Read the model definition and answer for the solid it produces. Units are mm, in the model's axes. A direction names the side the tool comes from. Coordinates: 2 decimals unless noted, no trailing zeros. Write each loop counter-clockwise with the first axis right and the second up, starting at its lowest first coordinate (ties: lowest second). Pieces come first, ordered by that corner, then holes. Notation, with made-up numbers: (-38.5, 2.5) -> (6.5, 2.5) arc R27 cw to (6.5, 40.5) -> close; hole circle Ø8 at (39.25, 71). An arc over 180 degrees is marked (long way). One line per item, written item: value. Start each with the question number.
1. For faces 5 (the flat face through (-1, 44.45, 5)), 6 (the cylindrical face through (77.926, 0.711, 7.997)), determine the directions among +Z, -Z, +X, -X, +Y, -Y from which every point of the face is accessible in a straight line to the end or side of a thin tool.
2. Given P1, Ø2, axis at x = -15.5, z = 5.5, coming from the +Y side; P2, Ø1, axis at x = 61, z = 8, coming from the -Y side; P3, Ø2, axis at x = 12.5, y = 37, coming from the +Z side, each flat-ended and moving along its own axis, determine where each tip first touches the part or whether it passes through.
3. Find section C-C, the plane x = -7. Write down the section's boundary in (y, z) (3 decimals).
4. Find section A-A, the plane y = -42. Write down the section's boundary in (x, z) (3 decimals), and give its area (3 significant figures).
5. Find section B-B, the plane z = 6.75. Write down the section's boundary in (x, y) (3 decimals), and give its area (3 significant figures).
6. Consider line 1 along X through (y, z) = (-5, 5) (3 decimals); line 2 along X through (y, z) = (2, 2) (3 decimals); line 3 along Y through (x, z) = (-71.5, 1.5). Determine where each line is inside the solid, lowest interval first.
7. For a pull along Y with two mould halves and no side action, classify faces 1 (the flat face through (-79.375, -1, 2)), 2 (the flat face through (-1, -50.8, 2)), 3 (the flat face through (-1, -44.45, 5)), 4 (the flat face through (-1, 50.8, 2)) as pulls with the +Y half, pulls with the -Y half, needs draft (parallel to the pull), parting line crosses it, or undercut.
```python
from build123d import *

# Parameters (mm, degrees)
F0_W     = 158.75
F0_H     = 101.6
F0_W_2   = 146.05
F0_H_2   = 88.9
F1_DEPTH = 9.525
F2_R     = 5.08
F3_DEPTH = 1.27


with BuildPart() as f1:
    # F0 (on Top) → F1 (new body)
    with BuildSketch(Plane.XY):
        Rectangle(F0_W, F0_H)
        Rectangle(F0_W_2, F0_H_2, mode=Mode.SUBTRACT)
    extrude(amount=F1_DEPTH)

    # F2
    f2_edges = [f1.edges().sort_by_distance(p)[0] for p in [
        (-79.375, 0, 9.525),
        (0, -50.8, 9.525),
        (79.375, 0, 9.525),
        (0, 50.8, 9.525),
    ]]
    fillet(f2_edges, radius=F2_R)

    # F0 (on Top) → F3 (join)
    with BuildSketch(Plane.XY):
        Rectangle(F0_W_2, F0_H_2)
    extrude(amount=F3_DEPTH)


solid = f1.part
```
Answer block:
1. face 5: +Z
1. face 6: +Z, +X, +Y, -Y
2. P1: stops at y = 50.8
2. P2: stops at y = -49.78
2. P3: stops at z = 1.27
3. outline: (-50.8, 0) -> (50.8, 0) -> (50.8, 4.445) arc R5.08 ccw to (45.72, 9.525) -> (44.45, 9.525) -> (44.45, 1.27) -> (-44.45, 1.27) -> (-44.45, 9.525) -> (-45.72, 9.525) arc R5.08 ccw to (-50.8, 4.445) -> close
4. outline: (-79.375, 0) -> (79.375, 0) -> (79.375, 4.445) arc R5.08 ccw to (74.295, 9.525) -> (73.025, 9.525) -> (73.025, 1.27) -> (-73.025, 1.27) -> (-73.025, 9.525) -> (-74.295, 9.525) arc R5.08 ccw to (-79.375, 4.445) -> close
4. area: 295 mm2
5. outline: (-78.822, -50.247) -> (78.822, -50.247) -> (78.822, 50.247) -> (-78.822, 50.247) -> close; hole (-73.025, -44.45) -> (73.025, -44.45) -> (73.025, 44.45) -> (-73.025, 44.45) -> close
5. area: 2,860 mm2
6. line 1: x = -79.345 to -73.025, 73.025 to 79.345
6. line 2: x = -79.375 to -73.025, 73.025 to 79.375
6. line 3: y = -50.8 to -44.45, 44.45 to 50.8
7. face 1: needs draft
7. face 2: pulls with the -Y half
7. face 3: undercut
7. face 4: pulls with the +Y half
